Input: part model. Units: mm. Frame: model coordinates. Coordinates: 2 decimals unless noted, no trailing zeros. Order: outer loops, then holes, each group sorted by start corner. A loop starts at its lowest first (then second) coordinate and runs counter-clockwise, first axis right, second up. Notation, with made-up numbers: (47, 80) -> (78, 80) arc R16 ccw to (78, 97) -> close; hole circle Ø2 at (23, -10). An arc over 180 degrees is marked (long way). Write each question's results on one line, items separated by ' | '.
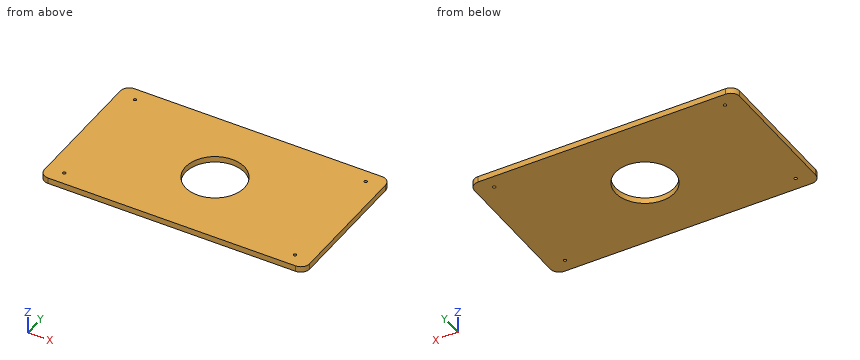
```python
from build123d import *

# Parameters (mm, degrees)
CROQUIS1_R              = 50
SALIENTE_EXTRUIR1_DEPTH = 10
CROQUIS2_R              = 2.5
CORTAR_EXTRUIR1_DEPTH   = 10


with BuildPart() as part:
    # Croquis1 → Saliente-Extruir1 (new body)
    with BuildSketch(Plane.XY):
        with BuildLine():
            Line((15, 0), (435, 0))
            ThreePointArc((435, 0), (445.606601718, 4.393398282), (450, 15))
            Line((450, 15), (450, 235))
            ThreePointArc((450, 235), (445.606601718, 245.606601718), (435, 250))
            Line((435, 250), (15, 250))
            ThreePointArc((15, 250), (4.393398282, 245.606601718), (0, 235))
            Line((0, 235), (0, 15))
            ThreePointArc((0, 15), (4.393398282, 4.393398282), (15, 0))
        make_face()
        with Locations((225, 125)):
            Circle(CROQUIS1_R, mode=Mode.SUBTRACT)
    extrude(amount=SALIENTE_EXTRUIR1_DEPTH)

    # Croquis2 → Cortar-Extruir1 (cut)
    with BuildSketch(Plane.XY.offset(10)):
        with Locations((420.681818182, 22.5)):
            Circle(CROQUIS2_R)
        with Locations((420.681818182, 227.5)):
            Circle(CROQUIS2_R)
        with Locations(Location((29.318181818, 227.5, 0), (0, 0, 180))):
            Circle(CROQUIS2_R)
        with Locations(Location((29.318181818, 22.5, 0), (0, 0, 180))):
            Circle(CROQUIS2_R)
    extrude(amount=-CORTAR_EXTRUIR1_DEPTH, mode=Mode.SUBTRACT)


solid = part.part
```
(1) Cut plane A-A, the plane x = 225. Return loops of the section in (y, z), plus the area to 3 significant figures.
Return value:
outline: (0, 0) -> (75, 0) -> (75, 10) -> (0, 10) -> close; (175, 0) -> (250, 0) -> (250, 10) -> (175, 10) -> close | area: 1,500 mm2
(2) Cut plane C-C, the plane z = 6.25. Return loops of the section in (x, y).
Return value:
outline: (0, 15) arc R15 ccw to (15, 0) -> (435, 0) arc R15 ccw to (450, 15) -> (450, 235) arc R15 ccw to (435, 250) -> (15, 250) arc R15 ccw to (0, 235) -> close; hole circle Ø5 at (29.32, 22.5); hole circle Ø5 at (29.32, 227.5); hole circle Ø100 at (225, 125); hole circle Ø5 at (420.68, 22.5); hole circle Ø5 at (420.68, 227.5)
(3) Cut plane B-B, the plane y = 155. Return loops of the section in (x, z).
Return value:
outline: (0, 0) -> (185, 0) -> (185, 10) -> (0, 10) -> close; (265, 0) -> (450, 0) -> (450, 10) -> (265, 10) -> close
(4) Line query: line 1 along X through (y, z) = (227.5, 7.5); line 2 along Y through (x, z) = (225, 6.75); line 3 along X through (y, z) = (157, 4.5). Output: solid intervals per line, ascending. Write a range as from..to.
Return value:
line 1: 0..26.82, 31.82..418.18, 423.18..450 | line 2: 0..75, 175..250 | line 3: 0..186.58, 263.42..450
(5) Pin query (flat end, axial travel): P1, Ø6, axis at x = 420.68, y = 227.5, coming from the -Z side. Return the tip coordinate at first contact, or that it passes through.
Return value:
P1: z = 0
